Geometry: see drawing. Coordinates: mm, zero at the bounding-box minimum. A direction names the side the tool comes from. Round coordinates to 2 decimals unless told otherwise and drop trailing zeros. Write each loop counter-clockwise with the first axis right and the second up, starting at its lowest first coordinate (ties: lowest second). Pieces come first, ordered by that corner, then holes.
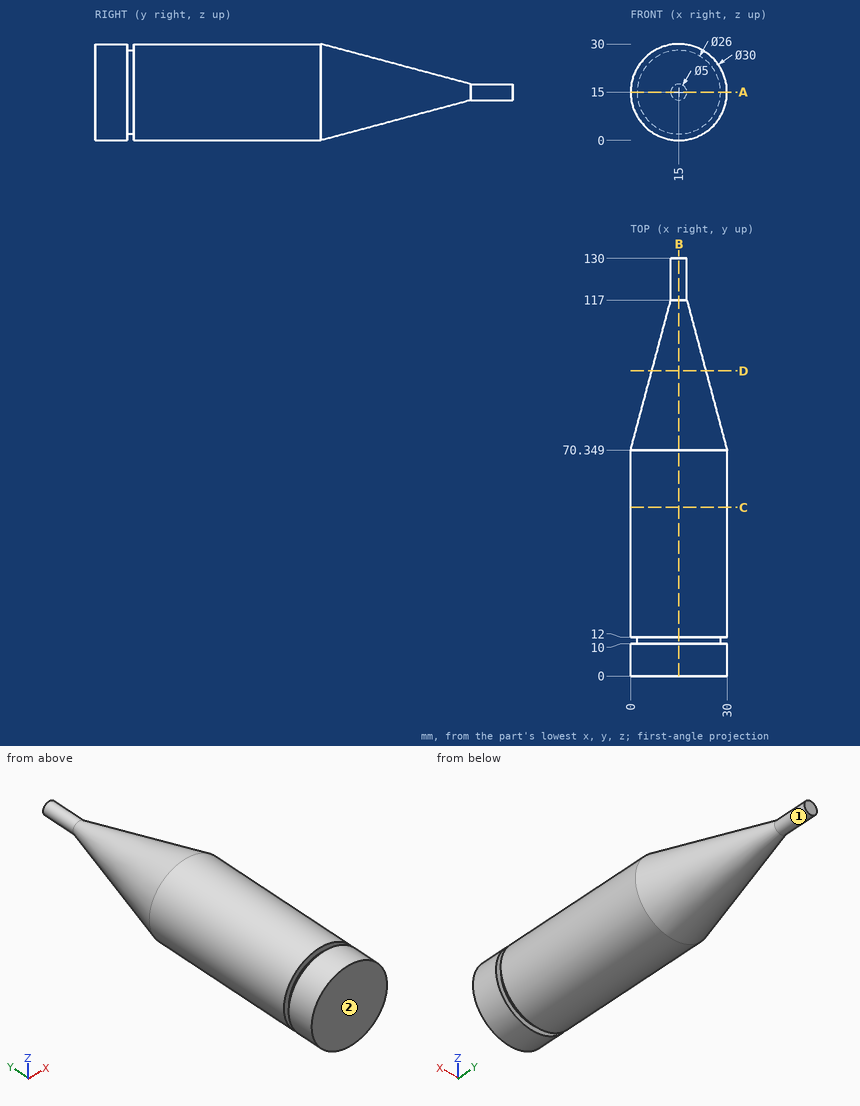
Q1. Section query C-C, the plane y = 52.5. Output: boundary loops of the cut face in (x, z), and give its area (3 significant figures).
Q2. Section query A-A, the plane z = 15. Output: boundary loops of the cut face in (x, y), and give its area (3 significant figures).
Q3. Set-up query: the marked faces 1 and 2. Return all of +Z, -Z, +X, -X, +Y, -Y with unobstructed straight access to the full face (end or side cutting, diameter ignored); none if empty.
Q4. Section query B-B, the plane x = 15. Output: boundary loops of the cut face in (y, z), and give its area (3 significant figures).
Q5. Section query D-D, the plane y = 95. Output: boundary loops of the cut face in (x, z) (1 decimal), and give its area (3 significant figures).
Q6. Line query: line 1 (Z direction, x = 14.5, y = 28.5); line 2 (X direction, y = 18, z = 15.25); line 3 (X direction, y = 32, z = 7.5). Output: solid intervals per line, ascending.
Q7. Pin query (flat end, axial travel): P1, Ø6, axis at y = 76.5, z = 22, coming from the +X side; P2, Ø4, axis at y = 36.5, z = 11, coming from the -X side; P3, Ø3, axis at x = 23.5, y = 80, coming from the -Z side. Return the tip coordinate at first contact, or that it passes through.
Filled in:
1. outline: circle Ø30 at (15, 15)
1. area: 707 mm2
2. outline: (0, 0) - (30, 0) - (30, 10) - (28, 10) - (28, 12) - (30, 12) - (30, 70.35) - (17.5, 117) - (17.5, 130) - (12.5, 130) - (12.5, 117) - (0, 70.35) - (0, 12) - (2, 12) - (2, 10) - (0, 10) - close
2. area: 2,980 mm2
3. face 1: +Y
3. face 2: +Z, -Z, +X, -X, -Y
4. outline: (0, 0) - (10, 0) - (10, 2) - (12, 2) - (12, 0) - (70.35, 0) - (117, 12.5) - (130, 12.5) - (130, 17.5) - (117, 17.5) - (70.35, 30) - (12, 30) - (12, 28) - (10, 28) - (10, 30) - (0, 30) - close
4. area: 2,980 mm2
5. outline: circle Ø16.8 at (15, 15)
5. area: 221 mm2
6. line 1: z = 0.01 to 29.99
6. line 2: x = 0 to 30
6. line 3: x = 2.01 to 27.99
7. P1: stops at x = 28.05
7. P2: stops at x = 0.13
7. P3: stops at z = 4.64
